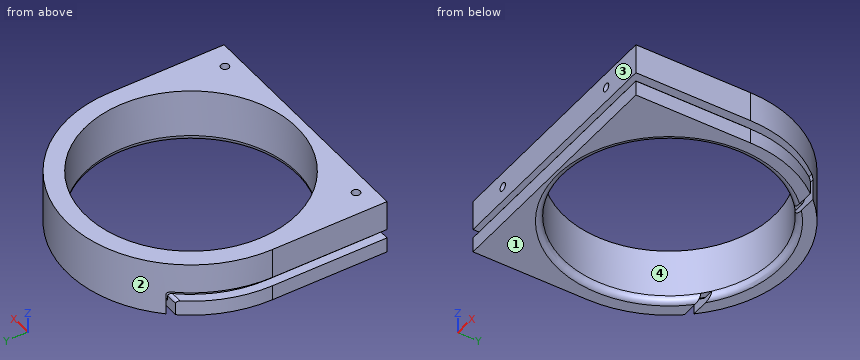
```python
from build123d import *

# Parameters (mm, degrees)
SKETCH_1_R                            = 35.00000000000001
EXTRUDE_21_DEPTH                      = 20
CUT_EXTRUDE_2_DEPTH                   = 4
CUT_EXTRUDE_3_DEPTH                   = 8
CUT_EXTRUDE_4_DEPTH                   = 1
CUT_EXTRUDE_4_DEPTH_BACK              = 2
FILLET_1_R                            = 1
SKETCH_8_W                            = 82
SKETCH_8_H                            = 2
CUT_EXTRUDE_5_DEPTH                   = 92.22499672787059
FILLET_3_R                            = 2
HOLE_WIZARD_2_7_2_7_1_D               = 2.7
HOLE_WIZARD_2_7_2_7_1_DEPTH           = 7
HOLE_WIZARD_2_7_2_7_1_TIP             = 0.8111618356872065
HOLE_WIZARD_2_7_2_7_1_ON_FACE_2_D     = 2.7
HOLE_WIZARD_2_7_2_7_1_ON_FACE_2_DEPTH = 7
HOLE_WIZARD_2_7_2_7_1_ON_FACE_2_TIP   = 0.8111618356872065


with BuildPart() as part:
    # 草图1 → 厚度21 (new body)
    with BuildSketch(Plane.XY):
        with BuildLine():
            Line((-41, 0), (-41, -38.00000000000001))
            Line((-41, -38.00000000000001), (41, -38.00000000000001))
            Line((41, -38.00000000000001), (41, 0))
            ThreePointArc((41, 0), (2.51e-15, 41), (-41, 0))
        make_face()
        Circle(SKETCH_1_R, mode=Mode.SUBTRACT)
    extrude(amount=EXTRUDE_21_DEPTH)

    # 草图5 → 切除-拉伸2 (cut)
    with BuildSketch(Plane(origin=(0, 0, 0), x_dir=(-1, 0, 0), z_dir=(0, 0, -1))):
        with BuildLine():
            Line((-21.000000000000004, 28.00000000000001), (-25.690465157330244, 28.000000000000007))
            ThreePointArc((-25.690465157330244, 28.000000000000007), (-26.720357920143798, 27.01892804349219), (-27.712812921102028, 26.00000000000001))
            Line((-27.712812921102028, 26.00000000000001), (-23.430749027719965, 26.000000000000007))
            ThreePointArc((-23.43074902771997, 26.000000000000007), (-22.237870059676574, 27.02734051306086), (-21.000000000000007, 28.00000000000001))
        make_face()
        with BuildLine():
            Line((25.690465157330244, 28.00000000000001), (20.99999999999999, 28.00000000000001))
            ThreePointArc((20.99999999999999, 28.000000000000014), (22.237870059676567, 27.027340513060857), (23.430749027719965, 26.000000000000007))
            Line((23.430749027719965, 26.000000000000007), (27.712812921102028, 26.00000000000001))
            ThreePointArc((27.712812921102035, 26.000000000000014), (26.720357920143798, 27.018928043492192), (25.69046515733025, 28.000000000000018))
        make_face()
    extrude(amount=-CUT_EXTRUDE_2_DEPTH, mode=Mode.SUBTRACT)

    # 草图6 → 切除-拉伸3 (cut)
    with BuildSketch(Plane(origin=(0, 0, 0), x_dir=(-1, 0, 0), z_dir=(0, 0, -1))):
        with BuildLine():
            ThreePointArc((-27.712812921102028, 26.000000000000004), (-26.72035792014379, 27.01892804349218), (-25.690465157330244, 28.00000000000001))
            Line((-25.690465157330244, 28.000000000000007), (-29.949958263743014, 28.000000000000007))
            ThreePointArc((-29.949958263743238, 28.00000000000068), (-30.842062505518594, 27.014203308735276), (-31.701734968294286, 26.000000000000522))
            Line((-31.70173496829411, 26.000000000000007), (-27.712812921102028, 26.000000000000004))
        make_face()
        with BuildLine():
            ThreePointArc((31.70173496829428, 26.00000000000053), (30.842062505518587, 27.01420330873528), (29.949958263743248, 28.000000000000668))
            Line((29.94995826374302, 28.000000000000007), (25.690465157330244, 28.000000000000007))
            ThreePointArc((25.690465157330244, 28.000000000000007), (26.720357920143798, 27.01892804349219), (27.712812921102028, 26.000000000000007))
            Line((27.712812921102028, 26.000000000000004), (31.701734968294097, 26.000000000000007))
        make_face()
        with BuildLine():
            Line((37.167004412093284, 28.000000000000007), (29.94995826374302, 28.000000000000007))
            ThreePointArc((29.949958263743248, 28.000000000000668), (30.842062505518587, 27.01420330873528), (31.70173496829428, 26.00000000000053))
            Line((31.701734968294097, 26.000000000000007), (37.167004412093284, 26.00000000000001))
            Line((37.167004412093284, 26.00000000000001), (37.167004412093284, 28.000000000000007))
        make_face()
        with BuildLine():
            ThreePointArc((-31.701734968294286, 26.000000000000522), (-30.842062505518594, 27.014203308735276), (-29.949958263743238, 28.00000000000068))
            Line((-29.949958263743014, 28.000000000000007), (-37.167004412093284, 28.000000000000007))
            Line((-37.167004412093284, 28.000000000000007), (-37.167004412093284, 26.00000000000001))
            Line((-37.167004412093284, 26.00000000000001), (-31.70173496829411, 26.000000000000007))
        make_face()
    extrude(amount=-CUT_EXTRUDE_3_DEPTH, mode=Mode.SUBTRACT)

    # 草图7 → 切除-拉伸4 (cut, two sides: drawn at the far end of the back side and taken through both)
    with BuildSketch(Plane(origin=(0, 0, 8), x_dir=(-1, 0, 0), z_dir=(0, 0, -1)).offset(-CUT_EXTRUDE_4_DEPTH_BACK)):
        with BuildLine():
            Line((-38, -36.00000000000001), (37.99999999999999, -36.00000000000001))
            Line((37.99999999999999, -36.00000000000001), (37.99999999999999, 0))
            ThreePointArc((37.99999999999999, 0), (34.786762395906784, 15.29317370628887), (25.690465157330244, 28.00000000000001))
            Line((25.690465157330244, 28.00000000000001), (29.949958263743873, 28.000000000000007))
            ThreePointArc((29.949958263743873, 28.000000000000007), (38.13756867455958, 15.050775913329202), (40.999999999999986, 0))
            Line((40.999999999999986, 0), (41, -38.00000000000001))
            Line((41, -38.00000000000001), (-41, -38.00000000000001))
            Line((-41, -38.00000000000001), (-40.999999999999986, 0))
            ThreePointArc((-40.999999999999986, 0), (-38.137568674559596, 15.050775913329224), (-29.949958263743873, 28.000000000000007))
            Line((-29.949958263743873, 28.000000000000007), (-25.69046515733023, 28.00000000000001))
            ThreePointArc((-25.69046515733023, 28.00000000000001), (-34.78676239590678, 15.293173706288876), (-37.99999999999999, 0))
            Line((-37.99999999999999, 0), (-38, -36.00000000000001))
        make_face()
    extrude(amount=CUT_EXTRUDE_4_DEPTH + CUT_EXTRUDE_4_DEPTH_BACK, mode=Mode.SUBTRACT)

    # 圆角1
    fillet_1_edges = [part.edges().sort_by_distance(p)[0] for p in [
        (29.707273944699274, 26.000000000000004, 7),
        (-29.707273944699253, 26.000000000000004, 7),
        (-37.99999999999999, -36.00000000000001, 8.5),
        (38, -36.00000000000001, 8.5),
        (-27.82021171053706, 28.000000000000007, 10),
        (27.820211710537052, 28.000000000000007, 10),
        (26.72035792014379, 27.01892804349218, 4),
        (-26.720357920143798, 27.018928043492195, 4),
    ]]
    fillet(fillet_1_edges, radius=FILLET_1_R)

    # 草图8 → 切除-拉伸5 (cut, through all)
    with BuildSketch(Plane.XZ.offset(38.00000000000001)):
        with Locations((0, 1)):
            Rectangle(SKETCH_8_W, SKETCH_8_H)
    extrude(amount=-CUT_EXTRUDE_5_DEPTH, mode=Mode.SUBTRACT)

    # 圆角3
    fillet_3_edges = [part.edges().sort_by_distance(p)[0] for p in [
        (-14.228910429646426, -31.97714977894527, 2),
        (-6.43e-15, 35.00000000000001, 2),
    ]]
    fillet(fillet_3_edges, radius=FILLET_3_R)

    # Ø2.7 (2.7) 直径孔1
    with Locations(Plane(origin=(-33, -33, 20), x_dir=(1, 0, 0), z_dir=(0, 0, 1))):
        with Locations((0, 0), (66, 0)):
            Hole(HOLE_WIZARD_2_7_2_7_1_D / 2, depth=HOLE_WIZARD_2_7_2_7_1_DEPTH)
            with Locations((0, 0, -(HOLE_WIZARD_2_7_2_7_1_DEPTH + HOLE_WIZARD_2_7_2_7_1_TIP / 2))):  # 118° drill point
                Cone(0, HOLE_WIZARD_2_7_2_7_1_D / 2, HOLE_WIZARD_2_7_2_7_1_TIP, mode=Mode.SUBTRACT)

    # Ø2.7 (2.7) 直径孔1 on face 2
    with Locations(Plane(origin=(26, -38, 15), x_dir=(0, 0, -1), z_dir=(0, -1, 0))):
        with Locations((0, 0), (0, -52)):
            Hole(HOLE_WIZARD_2_7_2_7_1_ON_FACE_2_D / 2, depth=HOLE_WIZARD_2_7_2_7_1_ON_FACE_2_DEPTH)
            with Locations((0, 0, -(HOLE_WIZARD_2_7_2_7_1_ON_FACE_2_DEPTH + HOLE_WIZARD_2_7_2_7_1_ON_FACE_2_TIP / 2))):  # 118° drill point
                Cone(0, HOLE_WIZARD_2_7_2_7_1_ON_FACE_2_D / 2, HOLE_WIZARD_2_7_2_7_1_ON_FACE_2_TIP, mode=Mode.SUBTRACT)


solid = part.part
```
Build history of the part. All positions in model axes, mm. Face numbers are marked on the shaded views. Round coordinates to 2 decimals unless told otherwise and drop trailing zeros. Write each loop counter-clockwise with the first axis right and the second up, starting at its lowest first coordinate (ties: lowest second). Pieces come first, ordered by that corner, then holes.
1) Drill centre lines: probe 1 along X at (y, z) = (-36, 15); probe 2 along Z at (x, y) = (38, 13.5); probe 3 along Z at (x, y) = (-26, -34.5). Where is each one in solid material? Low to high.
2) Band-saw the part on B-B, the plane x = 0. List the corners of the cut face in (y, z).
3) Pin check, flat tips, straight feed: pin 1 (1 mm diameter, centred on x = 30.5, z = 17.5, fed in from +Y); pin 2 (3.5 mm diameter, centred on y = -14.5, z = 8, fed in from +X); pin 3 (1.2 mm diameter, centred on x = 29, z = 3, fed in from +Y); pin 4 (3.5 mm diameter, centred on x = -26, z = 15, fed in from +Y). Stop position of each tip, or through.
4) Band-saw the part on A-A, the plane z = 11. List the corners of the cut face in (x, y), and give its area (3 significant figures).
5) Mould opens along Y. For the marked faces 1, 2, 3 and 4 say: +Y half, -Y half, draft (parallel to the pull), parting line (faces both ways), or undercut.
Ans:
1. probe 1: x = -41 to -27.35, -24.65 to 24.65, 27.35 to 41
1. probe 2: z = 2 to 7, 10 to 20
1. probe 3: z = 2 to 13.65, 16.35 to 20
2. outline: (-38, 2) - (-37, 2) arc R2 ccw to (-35, 4) - (-35, 20) - (-38, 20) - (-38, 10) - (-36, 10) - (-36, 7) - (-38, 7) - close; (35, 4) arc R2 ccw to (37, 2) - (41, 2) - (41, 20) - (35, 20) - close
3. pin 1: stops at y = 27.95
3. pin 2: stops at x = 41
3. pin 3: stops at y = 29.57
3. pin 4: stops at y = 33.06
4. outline: (-41, -38) - (41, -38) - (41, 0) arc R41 ccw to (-41, 0) - close; hole circle Ø70 at (0, 0)
4. area: 1,910 mm2
5. face 1: draft
5. face 2: +Y half
5. face 3: -Y half
5. face 4: undercut
